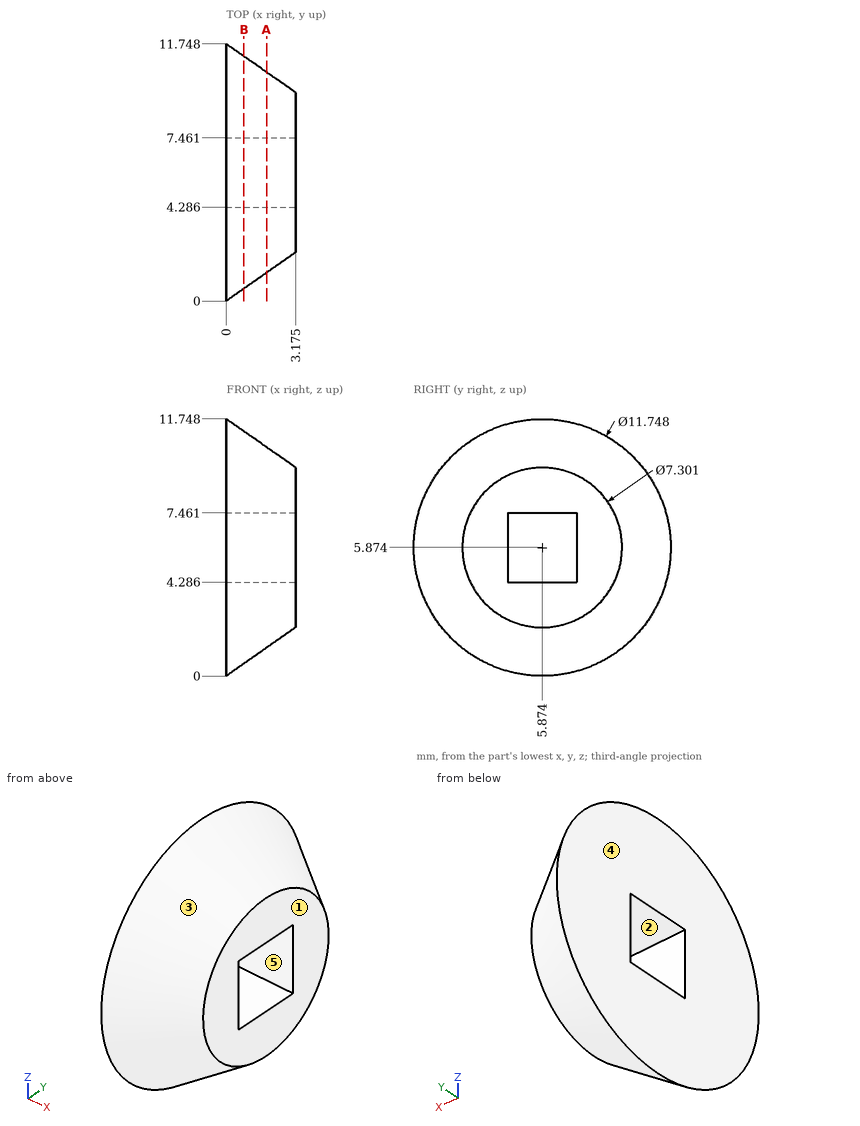
Part print with two shaded views. Sizes in mm from the minimum x, y, z corner. A direction names the side the tool comes from. Round coordinates to 2 decimals unless told otherwise and drop trailing zeros. Order: outer loops, then holes, each group sorted by start corner. A loop starts at its lowest first (then second) coordinate and runs counter-clockwise, first axis right, second up. Notation, with made-up numbers: M 49,84.5 L 54,84.5 A6 cw 54,93.5 Z; hole C 82,-23 d11. An arc over 180 degrees is marked long. Put each result on its own line as item: value. Start each with the question number.
1. Drill centre lines: probe 1 along Z at (x, y) = (2.75, 4.5) (1 decimal); probe 2 along Z at (x, y) = (0.25, 6.75) (1 decimal); probe 3 along Y at (x, z) = (1.1, 6.5) (1 decimal). Where is each one in solid material? Low to high. Write a range as [from, to].
2. Slice it at B-B on x = 0.8. List the corners of the cut face in (y, z).
3. Tool access for the marked faces 4 and 5: list every direction of +Z, -Z, +X, -X, +Y, -Y with a clear straight run to the whole face (end or side of a thin tool).
4. Drop flat-ended pins along their axis: pin 1 (3 mm diameter, centred on y = 3.5, z = 6, fed in from -X); pin 2 (1.5 mm diameter, centred on x = 2, y = 6, fed in from -Z) (1 decimal); pin 3 (1.6 mm diameter, centred on x = 1, z = 5.5, fed in from +Y); pin 4 (1 mm diameter, centred on x = 1.5, y = 6.5, fed in from +Z) (1 decimal). Give the stop position or say it passes through.
5. Two-plate mould, pull along Z, no slides. Class the marked faces 1, 2 and 3: +Z half, -Z half, draft (parallel to the pull), parting line (faces both ways), or undercut.
6. Slice it at A-A on x = 1.85. List the corners of the cut face in (y, z).
Findings:
1. probe 1: [2.2, 4.3], [7.5, 9.6]
1. probe 2: [0.2, 4.3], [7.5, 11.5]
1. probe 3: [0.8, 4.3], [7.5, 10.9]
2. outline: C 5.87,5.87 d10.63; hole M 4.29,4.29 L 7.46,4.29 L 7.46,7.46 L 4.29,7.46 Z
3. face 4: +Z, -Z, -X, +Y, -Y
3. face 5: +X, -X
4. pin 1: x = 0
4. pin 2: z = 0.9
4. pin 3: y = 11.6
4. pin 4: z = 11
5. face 1: draft
5. face 2: undercut
5. face 3: parting line
6. outline: C 5.87,5.87 d9.16; hole M 4.29,4.29 L 7.46,4.29 L 7.46,7.46 L 4.29,7.46 Z
